from build123d import *

# Parameters (mm, degrees)
F0_R            = 76.2
F0_R_2          = 4
F1_DEPTH        = 9.525
F3_D            = 6.35
F3_COPIES_COUNT = 20


# Not quite as in the source:
# - a pattern or mirror of a feature is missing from the dataset's text; its kind, count and spacing are read off the source's solid


with BuildPart() as f1:
    # F0 (on Top) → F1 (new body)
    with BuildSketch(Plane.XY):
        Circle(F0_R)
        Circle(F0_R_2, mode=Mode.SUBTRACT)
    extrude(amount=F1_DEPTH)

    # F3 (through all)
    with Locations(Plane.XY.offset(9.525)):
        with Locations((0, 69.85)):
            f3 = Hole(F3_D / 2)

    # F3_copies: F3 ×20 about axis
    f3_copies_axis = Axis((0, 0, 0), (0, 0, 1))
    for i in range(1, F3_COPIES_COUNT):
        add(f3.rotate(f3_copies_axis, i * 360 / F3_COPIES_COUNT), mode=Mode.SUBTRACT)


solid = f1.part
Design review of the part built by this model. Coordinates are the model's own, in mm. Round coordinates to 2 decimals unless told otherwise and drop trailing zeros. Write each loop counter-clockwise with the first axis right and the second up, starting at its lowest first coordinate (ties: lowest second). Pieces come first, ordered by that corner, then holes.
Item 1: Consider section B-B on z = 3.75. Count the separate pieces of the cut face and the enclosed holes in it, and give its area (3 significant figures).
Item 2: Consider section A-A on x = 0. Give the boundary of the cut face in (y, z) (3 decimals), and give its area (3 significant figures).
Item 3: Wall thickness on L1, parallel to Y at x = 0, z = 6.5 (3 decimals); L2, parallel to X at y = 55, z = 6; L3, parallel to Y at x = -58, z = 0.5: over which ranges is each line inside the solid? List them lowest first.
Item 4: Consider section C-C on x = -21. Give the boundary of the cut face in (y, z) (3 decimals).
Item 5: Consider section D-D on y = -29.5. Give the boundary of the cut face in (x, z) (3 decimals), and give its area (3 significant figures).
Item 6: For pin 1 Ø3 at (x, z) = (-35.5, 4) entering from +Y; pin 2 Ø2 at (x, z) = (49.5, 2.5) entering from +Y; pin 3 Ø4 at (x, z) = (-59.5, 4) entering from -Y, all flat-tipped, find the tip position at first contact; note any pin that passes through.
Item 7: Draft analysis for pull direction Y (two halves, no side actions). For faces 1 (the flat face through (16, 1, 9.525)), 2 (the cylindrical face through (-60.47, -46.367, 4.696)), 3 (the cylindrical face through (-55.501, -44.067, 4.696)), 4 (the cylindrical face through (0.69, 66.75, 4.7)), state which applies: released by +Y, released by -Y, zero draft, split by the parting line, or undercut.
Check values:
1. separate pieces: 1
1. enclosed holes: 21
1. area: 17,600 mm2
2. outline: (-76.2, 0) - (-73.025, 0) - (-73.025, 9.525) - (-76.2, 9.525) - close; (-66.675, 0) - (-4, 0) - (-4, 9.525) - (-66.675, 9.525) - close; (4, 0) - (66.675, 0) - (66.675, 9.525) - (4, 9.525) - close; (73.025, 0) - (76.2, 0) - (76.2, 9.525) - (73.025, 9.525) - close
2. area: 1,250 mm2
3. L1: y = -76.2 to -73.025, -66.675 to -4, 4 to 66.675, 73.025 to 76.2
3. L2: x = -52.74 to -43.85, -38.26 to 38.26, 43.85 to 52.74
3. L3: y = -49.42 to -43.86, -38.25 to 38.25, 43.86 to 49.42
4. outline: (-73.249, 0) - (-69.552, 0) - (-69.552, 9.525) - (-73.249, 9.525) - close; (-63.311, 0) - (63.311, 0) - (63.311, 9.525) - (-63.311, 9.525) - close; (69.552, 0) - (73.249, 0) - (73.249, 9.525) - (69.552, 9.525) - close
5. outline: (-70.258, 0) - (70.258, 0) - (70.258, 9.525) - (-70.258, 9.525) - close
5. area: 1,340 mm2
6. pin 1: stops at y = 68.19
6. pin 2: stops at y = 58.77
6. pin 3: stops at y = -50
7. face 1: zero draft
7. face 2: split by the parting line
7. face 3: undercut
7. face 4: undercut
